from build123d import *

# Parameters (mm, degrees)
SKETCH1_R           = 11
SKETCH1_R_2         = 1.5
BOSS_EXTRUDE1_DEPTH = 3
BOSS_EXTRUDE2_DEPTH = 3.175


with BuildPart() as part:
    # Sketch1 → Boss-Extrude1 (new body)
    with BuildSketch(Plane(origin=(0, 0, 0), x_dir=(1, 0, 0), z_dir=(0, 1, 0))):
        Polygon((20.42, -21), (-20.42, -21), (-25.5, -15.92), (-25.5, 30), (25.5, 30), (25.5, -15.92), align=None)
        Circle(SKETCH1_R, mode=Mode.SUBTRACT)
        with Locations((15.5, -15.5)):
            Circle(SKETCH1_R_2, mode=Mode.SUBTRACT)
        with Locations((-15.5, -15.5)):
            Circle(SKETCH1_R_2, mode=Mode.SUBTRACT)
        with Locations((-15.5, 15.5)):
            Circle(SKETCH1_R_2, mode=Mode.SUBTRACT)
        with Locations((15.5, 15.5)):
            Circle(SKETCH1_R_2, mode=Mode.SUBTRACT)
    extrude(amount=BOSS_EXTRUDE1_DEPTH)

    # Sketch2 → Boss-Extrude2 (add)
    with BuildSketch(Plane.XY.offset(-30)):
        Polygon((-25.5, 0), (25.5, 0), (25.5, 43.18), (20.42, 48.26), (-20.42, 48.26), (-25.5, 43.18), align=None)
        with BuildLine():
            Line((-17.165, 40.11), (-17.165, 10.41))
            ThreePointArc((-17.165, 10.41), (-15.015, 8.26), (-12.865, 10.41))
            Line((-12.865, 10.41), (-12.865, 40.11))
            ThreePointArc((-12.865, 40.11), (-15.015, 42.26), (-17.165, 40.11))
        make_face(mode=Mode.SUBTRACT)
        with BuildLine():
            Line((12.865, 40.11), (12.865, 10.41))
            ThreePointArc((12.865, 10.41), (15.015, 8.26), (17.165, 10.41))
            Line((17.165, 10.41), (17.165, 40.11))
            ThreePointArc((17.165, 40.11), (15.015, 42.26), (12.865, 40.11))
        make_face(mode=Mode.SUBTRACT)
    extrude(amount=BOSS_EXTRUDE2_DEPTH)


solid = part.part
Check sheet for the modelled part. Datum: model origin and axes. Units: mm. A direction names the side the tool comes from. Coordinates: 2 decimals unless noted, no trailing zeros. Write each loop counter-clockwise with the first axis right and the second up, starting at its lowest first coordinate (ties: lowest second). Pieces come first, ordered by that corner, then holes. Notation, with made-up numbers: M -30,43 L -23,43 A6 cw -23,51 Z; hole C -5,15.5 d11. An arc over 180 degrees is marked long. Answer as CSV lines item,"result".
Q1. Mould release check, pull along Y, two halves, no side actions. Record for faces 4 (the face through (0, 24, -30)), 5 (the face through (14.97, 8.26, -28.43)), 6 (the face through (0, 3, -14)), 7 (the face through (12.865, 25, -28)): released by +Y, released by -Y, zero draft, split by the parting line, or undercut.
Check result:
face 4,"zero draft"
face 5,"undercut"
face 6,"released by +Y"
face 7,"undercut"
Q2. Cross-section at B-B (z = 0). Record the boundary of the cut face in (x, y).
Check result:
outline,"M -25.5,0 L -11,0 L -11,3 L -25.5,3 Z; M 11,0 L 25.5,0 L 25.5,3 L 11,3 Z"
Q3. Material ranges on probe 1 along X at (y, z) = (0.95, -15.5); probe 2 along Z at (x, y) = (0, 1); probe 3 along X at (y, z) = (2, 15), recorded low to high. Write a range as from..to.
Check result:
probe 1,"-25.5..-17, -14..14, 17..25.5"
probe 2,"-30..-11, 11..21"
probe 3,"-25.5..-16.91, -14.09..14.09, 16.91..25.5"
Q4. Go/stop test with flat-tipped pins: pin 1 (8 mm diameter, centred on x = 10, z = -20, fed in from +Y); pin 2 (22.5 mm diameter, centred on x = 9.5, y = 25, fed in from +Z) (3 decimals). Record where each tip stops, or that it passes through.
Check result:
pin 1,"y = 3"
pin 2,"z = -26.825"
Q5. Set-up check for faces 1 (the face through (23, 1.48, 18.42)), 2 (the face through (-15.06, 8.26, -28.43)), 3 (the face through (0, 26, -26.825)): record each of +Z, -Z, +X, -X, +Y, -Y from which the full face is reachable in a straight line by a thin tool's end or side.
Check result:
face 1,"+Z, +X, +Y, -Y"
face 2,"+Z, -Z"
face 3,"+Z, +X, -X, +Y"
Q6. Cross-section at C-C (x = 0). Record the boundary of the cut face in (y, z) (3 decimals), then the cut area to 3 significant figures.
Check result:
outline,"M 0,-30 L 48.26,-30 L 48.26,-26.825 L 3,-26.825 L 3,-11 L 0,-11 Z; M 0,11 L 3,11 L 3,21 L 0,21 Z"
area,"231 mm^2"
Q7. Cross-section at A-A (y = 15). Record the boundary of the cut face in (x, z) (3 decimals).
Check result:
outline,"M -25.5,-30 L -17.165,-30 L -17.165,-26.825 L -25.5,-26.825 Z; M -12.865,-30 L 12.865,-30 L 12.865,-26.825 L -12.865,-26.825 Z; M 17.165,-30 L 25.5,-30 L 25.5,-26.825 L 17.165,-26.825 Z"
Q8. Cross-section at D-D (x = -15.5). Record the boundary of the cut face in (y, z) (3 decimals).
Check result:
outline,"M 0,-30 L 8.315,-30 L 8.315,-26.825 L 3,-26.825 L 3,-17 L 0,-17 Z; M 0,-14 L 3,-14 L 3,14 L 0,14 Z; M 0,17 L 3,17 L 3,21 L 0,21 Z; M 42.205,-30 L 48.26,-30 L 48.26,-26.825 L 42.205,-26.825 Z"
